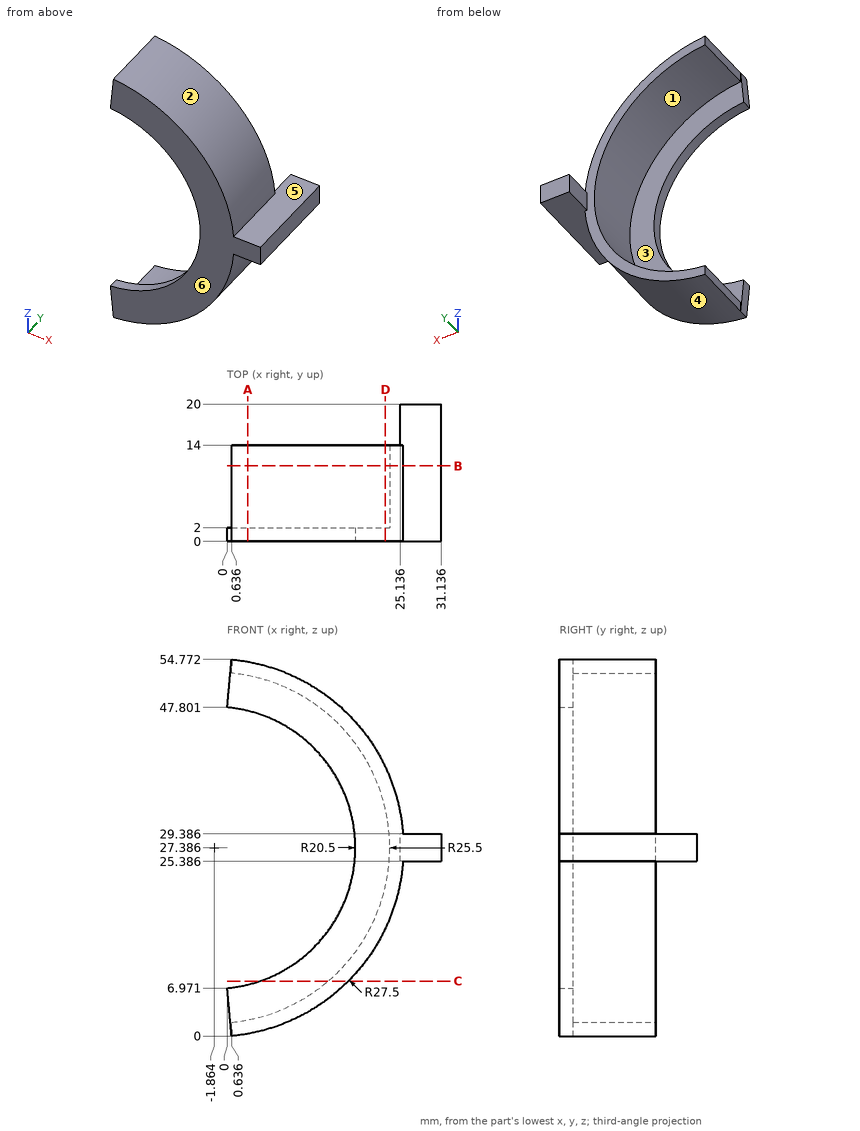
Study the drawing (mm; zero at the part's minimum x, y, z) and answer. A direction names the side the tool comes from. Give positions to 0.01 mm unless a question says otherwise; leave off trailing zeros. Write each loop counter-clockwise with the first axis right and the second up, starting at its lowest first coordinate (ties: lowest second). Pieces come first, ordered by that corner, then holes.
(1) The mould has two halves that part along Z. Classify the marked faces 3, 4, 5 and 6: pulls with the +Z half, pulls with the -Z half, needs draft (parallel to the pull), parting line crosses it, or undercut.
Final values:
face 3: undercut
face 4: pulls with the -Z half
face 5: pulls with the +Z half
face 6: needs draft
(2) The part is cut by section B-B on y = 11. Write down the section's boundary in (x, z).
Final values:
outline: (0.64, 0) arc R27.5 ccw to (25.56, 25.39) - (31.14, 25.39) - (31.14, 29.39) - (25.56, 29.39) arc R27.5 ccw to (0.64, 54.77) - (0.64, 52.76) arc R25.5 cw to (0.64, 2.01) - close
(3) Flat-ended cylindrical pins translate along their axes: pin 1 Ø3 at (x, y) = (28, 13) entering from -Z; pin 2 Ø7 at (x, z) = (12, 35) entering from +Y; pin 3 Ø2 at (y, z) = (18, 27) entering from -X; pin 4 Ø8 at (y, z) = (8.5, 19) entering from -X. Find the tip coordinate at first contact, or state that the pin passes through.
Final values:
pin 1: stops at z = 25.39
pin 2: passes through
pin 3: stops at x = 25.14
pin 4: stops at x = 20.43
(4) The part is cut by section A-A on x = 3. Write down the section's boundary in (y, z).
Final values:
outline: (0, 0.32) - (14, 0.32) - (14, 2.35) - (2, 2.35) - (2, 7.47) - (0, 7.47) - close; (0, 47.3) - (2, 47.3) - (2, 52.42) - (14, 52.42) - (14, 54.45) - (0, 54.45) - close
(5) The part is cut by section C-C on z = 8. Write down the section's boundary in (x, y).
Final values:
outline: (4.8, 0) - (17.64, 0) - (17.64, 14) - (14.7, 14) - (14.7, 2) - (4.8, 2) - close
(6) Which of the six approach directions +Z, -Z, +X, -X, +Y, -Y give full straight-line access (tool end or side, diameter ignored) to the marked faces 1 and 2?
Final values:
face 1: -X, +Y
face 2: +Z, +X, +Y, -Y
(7) The part is cut by section D-D on x = 23. Write down the section's boundary in (y, z) (1 decimal), plus the area to 3 significant figures.
Final values:
outline: (0, 15.6) - (14, 15.6) - (14, 21.7) - (2, 21.7) - (2, 33) - (14, 33) - (14, 39.1) - (0, 39.1) - close
area: 193 mm2
(8) Straight lines are drawn through the part: line 1 (Z direction, x = 28, y = 17.5); line 2 (Y direction, x = 6, z = 51.5); line 3 (Z direction, x = 21, y = 3.5) (1 decimal). For each, find the intervals that lie inside material, in ascending order.
Final values:
line 1: z = 25.39 to 29.39
line 2: y = 0 to 2
line 3: z = 12.1 to 16.1, 38.7 to 42.7
